```python
from build123d import *

# Parameters (mm, degrees)
F1_DEPTH = 1.2
F2_R     = 0.75
F3_DEPTH = 3
F7_DEPTH = 18


# Not quite as in the source:
# - an extrude ends at something that could not be found from the text; its depth is read off the source's solid


with BuildPart() as f1:
    # F0 (on Top) → F1 (new body)
    with BuildSketch(Plane.XY):
        with BuildLine():
            ThreePointArc((-0.75, -0.6614378278), (0, 1), (0.75, -0.6614378278))
            Line((0.75, -0.6614378278), (1, -5.4083269132))
            ThreePointArc((1, -5.4083269132), (1.7779895069, -5.7793923244), (2.5559790138, -5.4083269132))
            Line((2.5559790138, -5.4083269132), (3.5, -4.2426406871))
            ThreePointArc((3.5, -4.2426406871), (0, 5.5), (-3.5, -4.2426406871))
            Line((-3.5, -4.2426406871), (-2.5559790138, -5.4083269132))
            ThreePointArc((-2.5559790138, -5.4083269132), (-1.7779895069, -5.7793923244), (-1, -5.4083269132))
            Line((-1, -5.4083269132), (-0.75, -0.6614378278))
        make_face()
    extrude(amount=F1_DEPTH)

    # F2 (on Top) → F3 (join)
    with BuildSketch(Plane.XY):
        with Locations((-3, 1)):
            Circle(F2_R)
        with Locations((3, 1)):
            Circle(F2_R)
    extrude(amount=-F3_DEPTH)

    # F6 (on 3pt) → F7 (cut, through all)
    with BuildSketch(Plane(origin=(0, -0.105069468, 1.2468827773), x_dir=(1, 0, 0), z_dir=(0, -0.0839681251, 0.996468441))):
        Polygon((0.75, -0.558340171), (-0.75, -0.558340171), (-5.460082417, -0.558340171), (-5.460082417, -5.9262430295), (5.460082417, -5.9262430295), (5.460082417, -0.558340171), align=None)
    extrude(amount=F7_DEPTH, mode=Mode.SUBTRACT)


solid = f1.part
```
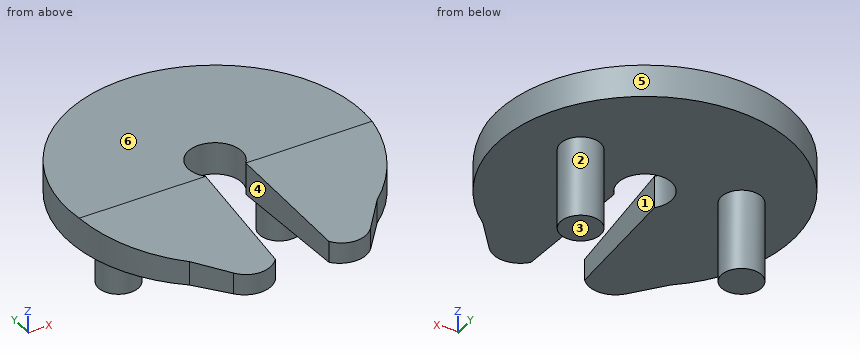
Verification items for the finished model (mm, model axes). Face numbers are marked on the shaded views. A direction names the side the tool comes from. Give positions to 0.01 mm unless a question says otherwise; leave off trailing zeros. Order: outer loops, then holes, each group sorted by start corner. A loop starts at its lowest first (then second) coordinate and runs counter-clockwise, first axis right, second up. Notation, with made-up numbers: (27, 82) -> (43, 82) arc R26 ccw to (43, 98) -> close; hole circle Ø7 at (56.5, -3). An arc over 180 degrees is marked (long way). One line per item, written item: value.
(1) Sectioned sample at B-B on z = 0.15. Record the cut outline in (x, y), then the cut area to 3 significant figures.
Final values:
outline: (-3.5, -4.24) -> (-2.56, -5.41) arc R1 ccw to (-1, -5.41) -> (-0.75, -0.66) arc R1 cw (long way) to (0.75, -0.66) -> (1, -5.41) arc R1 ccw to (2.56, -5.41) -> (3.5, -4.24) arc R5.5 ccw (long way) to start
area: 85.8 mm^2
(2) Tool access check on the marked faces 1, 2 and 3. Record the directions out of +Z, -Z, +X, -X, +Y, -Y that give a thin tool (end or side, any length) a straight path to the whole face; none if there is none.
Final values:
face 1: +Z, -Z, -Y
face 2: -Z
face 3: -Z, +X, -X, +Y, -Y
(3) Sectioned sample at C-C on x = 3.25. Record the cut outline in (y, z), then the cut area to 3 significant figures.
Final values:
outline: (-4.55, 0) -> (0.29, 0) -> (0.29, -3) -> (1.71, -3) -> (1.71, 0) -> (4.44, 0) -> (4.44, 1.2) -> (-0.66, 1.2) -> (-4.55, 0.87) -> close
area: 14.4 mm^2
(4) Scan lines: line 1 along X through (y, z) = (0, 0.5); line 2 along Z through (x, y) = (-3.25, 1.75); line 3 along Y through (x, z) = (0, 0.45). Record each from-to range of solid material in increasing order. Write a range as [from, to].
Final values:
line 1: [-5.5, -1], [1, 5.5]
line 2: [0, 1.2]
line 3: [1, 5.5]
(5) Sectioned sample at A-A on y = 0. Record the cut outline in (x, z).
Final values:
outline: (-5.5, 0) -> (-1, 0) -> (-1, 1.2) -> (-5.5, 1.2) -> close; (1, 0) -> (5.5, 0) -> (5.5, 1.2) -> (1, 1.2) -> close
(6) Gauge pin test, flat ends, axial feed: pin 1 (2.5 mm diameter, centred on x = 0, y = 0, fed in from +Z); pin 2 (1.5 mm diameter, centred on x = -4, z = -2.5, fed in from -Y); pin 3 (1.5 mm diameter, centred on x = 2.5, y = -4, fed in from -Z). Record the tip position at first contact, or that the pin passes through.
Final values:
pin 1: z = 1.2
pin 2: y = 0.29
pin 3: z = 0
(7) Draft check along X on the marked faces 4, 5 and 6. Enter one of: pulls with the +X half, pulls with the -X half, needs draft (parallel to the pull), parting line crosses it, or undercut.
Final values:
face 4: undercut
face 5: parting line crosses it
face 6: needs draft
(8) Sectioned sample at D-D on z = -1.95. Record the cut outline in (x, y).
Final values:
outline: circle Ø1.5 at (-3, 1); circle Ø1.5 at (3, 1)
